from build123d import *

# Parameters (mm, degrees)
F2_R     = 15
F3_DEPTH = 19
F4_R     = 12.5
F5_DEPTH = 25
F6_R     = 1.5


with BuildPart() as f1:
    # F0 (on Front) → F1 (revolve)
    with BuildSketch(Plane.XZ):
        Polygon((0, 17.5), (0, 0), (60, 0), (60, 10), (75, 10), (75, 15), (72, 15), (72, 17.5), (67, 17.5), (67, 15), (50, 15), (5, 17.5), align=None)
    revolve(axis=Axis((30, 0, 0), (-1, 0, 0)))

    # F2 (on Front) → F3 (join)
    with BuildSketch(Plane.XZ):
        with Locations((17.5, 0)):
            Circle(F2_R)
    extrude(amount=F3_DEPTH)

    # F4 (on face) → F5 (cut)
    with BuildSketch(Plane.XZ.offset(19)):
        with Locations((17.5, 0)):
            Circle(F4_R)
    extrude(amount=-F5_DEPTH, mode=Mode.SUBTRACT)

    # F6
    f6_edges = [f1.edges().sort_by_distance(p)[0] for p in [
        (0, 0, -17.5),
        (67, 0, -17.5),
        (72, 0, -17.5),
        (2.5, -19, 0),
        (75, 0, -15),
    ]]
    fillet(f6_edges, radius=F6_R)


solid = f1.part
The model under review builds one solid part; all positions refer to its coordinate system, in mm. A direction names the side the tool comes from. Give positions to 0.01 mm unless a question says otherwise; leave off trailing zeros. Write each loop counter-clockwise with the first axis right and the second up, starting at its lowest first coordinate (ties: lowest second). Pieces come first, ordered by that corner, then holes.
1. Draft analysis for pull direction Y (two halves, no side actions). For faces 1 (the cylindrical face through (67.6, -9.76, -2.17)), 2 (the flat face through (17, 6, 0)), 3 (the flat face through (0, 0, 0)), state which applies: +Y half, -Y half, draft (parallel to the pull), parting line (faces both ways), or undercut.
2. For P1, Ø10, axis at x = 28, z = 11.5, coming from the -Y side; P2, Ø12, axis at x = 56, z = 11.5, coming from the -Y side; P3, Ø5, axis at x = 25.5, z = 3.5, coming from the -Y side; P4, Ø6, axis at x = 20, z = 6.5, coming from the +Y side, all flat-tipped, find the tip position at first contact; note any pin that passes through.
3. Wall thickness on L1, parallel to Y at x = 70.5, z = 0; L2, parallel to Z at x = 17.5, y = -10.25; L3, parallel to Y at x = 63, z = 0: over which ranges is each line inside the solid? List them lowest first.
4. Add section C-C, the plane x = 36. Write out the cut boundary in (y, z), plus the area to 3 significant figures.
5. Add section B-B, the plane x = 65. Write out the cut boundary in (y, z).
6. Add section D-D, the plane x = 43.5. Write out the cut boundary in (y, z).
7. Tool access review of faces 4 (the conical face through (32.185, 15.854, -2.082)), 5 (the flat face through (60, 0, 0)), 6 (the cylindrical face through (31.356, -15.768, -5.745)): name each direction out of +Z, -Z, +X, -X, +Y, -Y from which nothing blocks a thin tool from reaching the whole face with its end or side.
Worked answers:
1. face 1: undercut
1. face 2: -Y half
1. face 3: draft
2. P1: stops at y = -19
2. P2: stops at y = -13.96
2. P3: stops at y = 6
2. P4: stops at y = 16.32
3. L1: y = -17.5 to -10, 10 to 17.5
3. L2: z = -15 to -12.5, 12.5 to 15
3. L3: y = -15 to -10, 10 to 15
4. outline: circle Ø31.56 at (0, 0)
4. area: 782 mm2
5. outline: circle Ø30 at (0, 0); hole circle Ø20 at (0, 0)
6. outline: circle Ø30.72 at (0, 0)
7. face 4: none
7. face 5: +X
7. face 6: -Y
